CAD build for the part. Positions are in the model's coordinates, mm. Round coordinates to 2 decimals unless told otherwise and drop trailing zeros. Loops run counter-clockwise (first coordinate to the right, second up) from the corner with the lowest first, then second, coordinate; pieces in that order, holes last. Notation, with made-up numbers: M 61,28.5 L 70,28.5 A18 ccw 70,40.5 Z; hole C 59,38 d10. An arc over 180 degrees is marked long. One line per item, written item: value. Start each with the question number.
from build123d import *

# Parameters (mm, degrees)
SKETCH_1_W          = 36
SKETCH_1_H          = 36
EXTRUDE_1_DEPTH     = 11
FILLET_1_R          = 1
SKETCH_2_R          = 1.25
CUT_EXTRUDE_1_DEPTH = 36


with BuildPart() as part:
    # 草图1 → 凸台-拉伸1 (new body)
    with BuildSketch(Plane(origin=(0, 0, 0), x_dir=(0, 0, -1), z_dir=(1, 0, 0))):
        with Locations((-12.735278258, 9.396435054)):
            Rectangle(SKETCH_1_W, SKETCH_1_H)
    extrude(amount=EXTRUDE_1_DEPTH)

    # 圆角1
    fillet_1_edges = [part.edges().sort_by_distance(p)[0] for p in [
        (11, 9.396435054, -5.264721742),
        (11, 27.396435054, 12.735278258),
        (11, 9.396435054, 30.735278258),
        (0, 27.396435054, 12.735278258),
        (0, 9.396435054, -5.264721742),
        (0, -8.603564946, 12.735278258),
        (0, 9.396435054, 30.735278258),
        (5.5, 27.396435054, 30.735278258),
        (5.5, 27.396435054, -5.264721742),
        (5.5, -8.603564946, -5.264721742),
        (5.5, -8.603564946, 30.735278258),
        (11, -8.603564946, 12.735278258),
    ]]
    fillet(fillet_1_edges, radius=FILLET_1_R)

    # 草图2 → 切除-拉伸1 (cut)
    with BuildSketch(Plane.XZ.offset(8.603564946)):
        with Locations(Location((5.5, 12.735278258, 0), (0, 0, 270))):
            Circle(SKETCH_2_R)
    extrude(amount=-CUT_EXTRUDE_1_DEPTH, mode=Mode.SUBTRACT)


solid = part.part
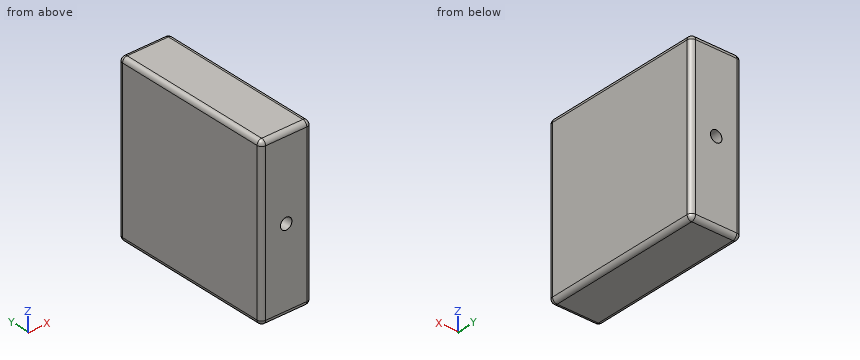
(1) Slice it at A-A, the plane x = 5.5. List the corners of the cut face in (y, z).
(2) Probe L1, parallel to Z at x = 6.5, y = 14; L2, parallel to Z at x = 6.25, y = 1; L3, parallel to Y at x = 10.75, z = 28.5 (3 decimals). List the from-to ranges inside material, lowest first.
(3) Flat gauge pin, fed straight in: P1, Ø2, axis at x = 5.5, z = 12.74, coming from the -Y side. Where does the tip first touch, or does it go through?
Check result:
1. outline: M -8.6,-4.26 A1 ccw -7.6,-5.26 L 26.4,-5.26 A1 ccw 27.4,-4.26 L 27.4,11.49 L -8.6,11.49 Z; M -8.6,13.99 L 27.4,13.99 L 27.4,29.74 A1 ccw 26.4,30.74 L -7.6,30.74 A1 ccw -8.6,29.74 Z
2. L1: z = -5.26 to 11.99, 13.49 to 30.74
2. L2: z = -5.26 to 11.74, 13.74 to 30.74
2. L3: y = -8.265 to 27.058
3. P1: passes through
